from build123d import *

# Parameters (mm, degrees)
F1_DEPTH = 76.2
F2_DEPTH = 63.5
F3_DEPTH = 12.7
F0_R     = 40.64
F4_DEPTH = 76.2
F5_DEPTH = 76.201
F6_DEPTH = 25.4
F7_DEPTH = 76.2
F8_DEPTH = 82.55
F9_DEPTH = 12.7


with BuildPart() as f1:
    # F0 (on Top) → F1 (new body, symmetric)
    with BuildSketch(Plane.XY):
        Polygon((324.1035716087, 782.4552381913), (-324.1035716087, 782.4552381913), (-782.4552381913, 324.1035716087), (-782.4552381913, -324.1035716087), (-324.1035716087, -782.4552381913), (324.1035716087, -782.4552381913), (782.4552381913, -324.1035716087), (782.4552381913, 324.1035716087), align=None)
        Polygon((-306.2038256122, 739.2414286435), (-253.5827489128, 739.2414286435), (253.5827489128, 739.2414286435), (306.2038256122, 739.2414286435), (343.4125457797, 702.032708476), (702.032708476, 343.4125457797), (739.2414286435, 306.2038256122), (739.2414286435, 253.5827489128), (739.2414286435, -253.5827489128), (739.2414286435, -306.2038256122), (702.032708476, -343.4125457797), (343.4125457797, -702.032708476), (306.2038256122, -739.2414286435), (253.5827489128, -739.2414286435), (-253.5827489128, -739.2414286435), (-306.2038256122, -739.2414286435), (-343.4125457797, -702.032708476), (-702.032708476, -343.4125457797), (-739.2414286435, -306.2038256122), (-739.2414286435, -253.5827489128), (-739.2414286435, 253.5827489128), (-739.2414286435, 306.2038256122), (-702.032708476, 343.4125457797), (-343.4125457797, 702.032708476), align=None, mode=Mode.SUBTRACT)
    extrude(amount=F1_DEPTH, both=True)

    # F0 (on Top) → F2 (join, symmetric)
    with BuildSketch(Plane.XY):
        Polygon((-572.3912798325, 289.7133077901), (-289.7133077901, 572.3912798325), (-343.4125457797, 702.032708476), (-702.032708476, 343.4125457797), align=None)
        Polygon((-253.5827489128, 739.2414286435), (-199.8835109232, 609.6), (199.8835109232, 609.6), (253.5827489128, 739.2414286435), align=None)
        Polygon((343.4125457797, 702.032708476), (289.7133077901, 572.3912798325), (572.3912798325, 289.7133077901), (702.032708476, 343.4125457797), align=None)
        Polygon((-609.6, -199.8835109232), (-609.6, 199.8835109232), (-739.2414286435, 253.5827489128), (-739.2414286435, -253.5827489128), align=None)
        Polygon((739.2414286435, 253.5827489128), (609.6, 199.8835109232), (609.6, -199.8835109232), (739.2414286435, -253.5827489128), align=None)
        Polygon((702.032708476, -343.4125457797), (572.3912798325, -289.7133077901), (289.7133077901, -572.3912798325), (343.4125457797, -702.032708476), align=None)
        Polygon((199.8835109232, -609.6), (-199.8835109232, -609.6), (-253.5827489128, -739.2414286435), (253.5827489128, -739.2414286435), align=None)
        Polygon((-289.7133077901, -572.3912798325), (-572.3912798325, -289.7133077901), (-702.032708476, -343.4125457797), (-343.4125457797, -702.032708476), align=None)
    extrude(amount=F2_DEPTH, both=True)

    # F3 (add): faces of the model
    f3_faces = [f1.faces().sort_by_distance(p)[0] for p in [
        (478.6967193132, -478.6967193132, -63.5),
        (0, -676.9793927162, -63.5),
        (-478.6967193132, -478.6967193132, -63.5),
        (-676.9793927162, 0, -63.5),
        (-478.6967193132, 478.6967193132, -63.5),
        (0, 676.9793927162, -63.5),
        (478.6967193132, 478.6967193132, -63.5),
        (676.9793927162, 0, -63.5),
    ]]
    extrude(f3_faces, amount=F3_DEPTH)

    # F0 (on Top) → F4 (join, symmetric)
    with BuildSketch(Plane.XY):
        Polygon((-289.7133077901, 572.3912798325), (-252.5045876226, 609.6), (-199.8835109232, 609.6), (-253.5827489128, 739.2414286435), (-306.2038256122, 739.2414286435), (-343.4125457797, 702.032708476), align=None)
        with Locations((-279.3542066174, 674.4207143217)):
            Circle(F0_R, mode=Mode.SUBTRACT)
        Polygon((253.5827489128, 739.2414286435), (199.8835109232, 609.6), (252.5045876226, 609.6), (289.7133077901, 572.3912798325), (343.4125457797, 702.032708476), (306.2038256122, 739.2414286435), align=None)
        with Locations((279.3542066174, 674.4207143217)):
            Circle(F0_R, mode=Mode.SUBTRACT)
        Polygon((-609.6, 252.5045876226), (-572.3912798325, 289.7133077901), (-702.032708476, 343.4125457797), (-739.2414286435, 306.2038256122), (-739.2414286435, 253.5827489128), (-609.6, 199.8835109232), align=None)
        with Locations((-674.4207143217, 279.3542066174)):
            Circle(F0_R, mode=Mode.SUBTRACT)
        Polygon((-609.6, -252.5045876226), (-609.6, -199.8835109232), (-739.2414286435, -253.5827489128), (-739.2414286435, -306.2038256122), (-702.032708476, -343.4125457797), (-572.3912798325, -289.7133077901), align=None)
        with Locations((-674.4207143217, -279.3542066174)):
            Circle(F0_R, mode=Mode.SUBTRACT)
        Polygon((702.032708476, 343.4125457797), (572.3912798325, 289.7133077901), (609.6, 252.5045876226), (609.6, 199.8835109232), (739.2414286435, 253.5827489128), (739.2414286435, 306.2038256122), align=None)
        with Locations((674.4207143217, 279.3542066174)):
            Circle(F0_R, mode=Mode.SUBTRACT)
        Polygon((739.2414286435, -253.5827489128), (609.6, -199.8835109232), (609.6, -252.5045876226), (572.3912798325, -289.7133077901), (702.032708476, -343.4125457797), (739.2414286435, -306.2038256122), align=None)
        with Locations((674.4207143217, -279.3542066174)):
            Circle(F0_R, mode=Mode.SUBTRACT)
        Polygon((-252.5045876226, -609.6), (-289.7133077901, -572.3912798325), (-343.4125457797, -702.032708476), (-306.2038256122, -739.2414286435), (-253.5827489128, -739.2414286435), (-199.8835109232, -609.6), align=None)
        with Locations((-279.3542066174, -674.4207143217)):
            Circle(F0_R, mode=Mode.SUBTRACT)
        Polygon((343.4125457797, -702.032708476), (289.7133077901, -572.3912798325), (252.5045876226, -609.6), (199.8835109232, -609.6), (253.5827489128, -739.2414286435), (306.2038256122, -739.2414286435), align=None)
        with Locations((279.3542066174, -674.4207143217)):
            Circle(F0_R, mode=Mode.SUBTRACT)
        with Locations((674.4207143217, 279.3542066174)):
            Circle(F0_R)
        with Locations((279.3542066174, 674.4207143217)):
            Circle(F0_R)
        with Locations((-279.3542066174, 674.4207143217)):
            Circle(F0_R)
        with Locations((-674.4207143217, 279.3542066174)):
            Circle(F0_R)
        with Locations((-674.4207143217, -279.3542066174)):
            Circle(F0_R)
        with Locations((-279.3542066174, -674.4207143217)):
            Circle(F0_R)
        with Locations((279.3542066174, -674.4207143217)):
            Circle(F0_R)
        with Locations((674.4207143217, -279.3542066174)):
            Circle(F0_R)
    extrude(amount=F4_DEPTH, both=True)

    # F0 (on Top) → F5 (cut, through all)
    with BuildSketch(Plane.XY):
        with Locations((-674.4207143217, 279.3542066174)):
            Circle(F0_R)
        with Locations((-279.3542066174, 674.4207143217)):
            Circle(F0_R)
        with Locations((279.3542066174, 674.4207143217)):
            Circle(F0_R)
        with Locations((674.4207143217, 279.3542066174)):
            Circle(F0_R)
        with Locations((674.4207143217, -279.3542066174)):
            Circle(F0_R)
        with Locations((279.3542066174, -674.4207143217)):
            Circle(F0_R)
        with Locations((-279.3542066174, -674.4207143217)):
            Circle(F0_R)
        with Locations((-674.4207143217, -279.3542066174)):
            Circle(F0_R)
    extrude(amount=F5_DEPTH, mode=Mode.SUBTRACT)

    # F0 (on Top) → F6 (join)
    with BuildSketch(Plane.XY):
        with Locations((-279.3542066174, 674.4207143217)):
            Circle(F0_R)
        with Locations((279.3542066174, 674.4207143217)):
            Circle(F0_R)
        with Locations((674.4207143217, 279.3542066174)):
            Circle(F0_R)
        with Locations((674.4207143217, -279.3542066174)):
            Circle(F0_R)
        with Locations((279.3542066174, -674.4207143217)):
            Circle(F0_R)
        with Locations((-279.3542066174, -674.4207143217)):
            Circle(F0_R)
        with Locations((-674.4207143217, -279.3542066174)):
            Circle(F0_R)
        with Locations((-674.4207143217, 279.3542066174)):
            Circle(F0_R)
    extrude(amount=F6_DEPTH)

    # F0 (on Top) → F7 (join)
    with BuildSketch(Plane.XY):
        Polygon((-199.8835109232, 609.6), (-252.5045876226, 609.6), (-289.7133077901, 572.3912798325), (-572.3912798325, 289.7133077901), (-609.6, 252.5045876226), (-609.6, 199.8835109232), (-609.6, -199.8835109232), (-609.6, -252.5045876226), (-572.3912798325, -289.7133077901), (-289.7133077901, -572.3912798325), (-252.5045876226, -609.6), (-199.8835109232, -609.6), (199.8835109232, -609.6), (252.5045876226, -609.6), (289.7133077901, -572.3912798325), (572.3912798325, -289.7133077901), (609.6, -252.5045876226), (609.6, -199.8835109232), (609.6, 199.8835109232), (609.6, 252.5045876226), (572.3912798325, 289.7133077901), (289.7133077901, 572.3912798325), (252.5045876226, 609.6), (199.8835109232, 609.6), align=None)
    extrude(amount=-F7_DEPTH)

    # F0 (on Top) → F8 (join)
    with BuildSketch(Plane.XY):
        Polygon((-199.8835109232, 609.6), (-252.5045876226, 609.6), (-289.7133077901, 572.3912798325), (-572.3912798325, 289.7133077901), (-609.6, 252.5045876226), (-609.6, 199.8835109232), (-609.6, -199.8835109232), (-609.6, -252.5045876226), (-572.3912798325, -289.7133077901), (-289.7133077901, -572.3912798325), (-252.5045876226, -609.6), (-199.8835109232, -609.6), (199.8835109232, -609.6), (252.5045876226, -609.6), (289.7133077901, -572.3912798325), (572.3912798325, -289.7133077901), (609.6, -252.5045876226), (609.6, -199.8835109232), (609.6, 199.8835109232), (609.6, 252.5045876226), (572.3912798325, 289.7133077901), (289.7133077901, 572.3912798325), (252.5045876226, 609.6), (199.8835109232, 609.6), align=None)
    extrude(amount=F8_DEPTH)

    # F9 (cut): faces of the model
    f9_faces = [f1.faces().sort_by_distance(p)[0] for p in [
        (0, -676.9793927162, 63.5),
        (478.6967193132, -478.6967193132, 63.5),
        (676.9793927162, 0, 63.5),
        (478.6967193132, 478.6967193132, 63.5),
        (0, 676.9793927162, 63.5),
        (-478.6967193132, 478.6967193132, 63.5),
        (-676.9793927162, 0, 63.5),
        (-478.6967193132, -478.6967193132, 63.5),
    ]]
    extrude(f9_faces, amount=-F9_DEPTH, mode=Mode.SUBTRACT)


solid = f1.part
Could you check a few things on this model? Use its own coordinates, in mm. Give positions to 0.01 mm unless a question says otherwise; leave off trailing zeros. Order: outer loops, then holes, each group sorted by start corner. A loop starts at its lowest first (then second) coordinate and runs counter-clockwise, first axis right, second up. Notation, with made-up numbers: (-13.75, 51.5) - (20.25, 51.5) arc R29 cw to (20.25, 71.5) - close; hole circle Ø10 at (18, 84). An arc over 180 degrees is marked (long way). Return JSON: item names as keys, results as strings. Group by question number.
Q1. Will these pins go through, and if not, where does the flat tip stop? pin 1 Ø1 at (y, z) = (-444, -38.5) entering from +X; pin 2 Ø12 at (x, y) = (-588, -442) entering from +Z; pin 3 Ø24.5 at (x, y) = (290.5, -671) entering from +Z.
Q2. Thinking about a two-plate mould opening in Y: for faces 1 (the face through (464, 482, 50.8)), 2 (the face through (-550.07, 556.49, 1.07)), which applies, pulls with the +Y half, pulls with the -Y half, needs draft (parallel to the pull), parting line crosses it, or undercut?
Q3. Please list where these lines run through material, in increasing order: line 1 along X through (y, z) = (6.5, 61.5); line 2 along X through (y, z) = (-573, 55). Write a range as [from, to].
Q4. Suppose I cut it at A-A, the plane y = -96.5. Please give me the cut outline in (x, z).
Q5. Suppose I cut it at B-B, the plane z = -24. Please give me the cut outline in (x, y), and give its area (3 significant figures).
Resolved:
{
 "1": {"pin 1": "stops at x = 663.06", "pin 2": "stops at z = 50.8", "pin 3": "stops at z = 25.4"},
 "2": {"face 1": "undercut", "face 2": "pulls with the +Y half"},
 "3": {"line 1": "x = [-782.46, -739.24], [-609.6, 609.6], [739.24, 782.46]", "line 2": "x = [-533.56, -472.45], [-289.97, 289.97], [472.45, 533.56]"},
 "4": {"outline": "(-782.46, -76.2) - (782.46, -76.2) - (782.46, 76.2) - (739.24, 76.2) - (739.24, 50.8) - (609.6, 50.8) - (609.6, 82.55) - (-609.6, 82.55) - (-609.6, 50.8) - (-739.24, 50.8) - (-739.24, 76.2) - (-782.46, 76.2) - close"},
 "5": {"outline": "(-782.46, -324.1) - (-324.1, -782.46) - (324.1, -782.46) - (782.46, -324.1) - (782.46, 324.1) - (324.1, 782.46) - (-324.1, 782.46) - (-782.46, 324.1) - close", "area": "2,030,000 mm2"}
}
